Build history of the part. All positions in model axes, mm. A direction names the side the tool comes from. Round coordinates to 2 decimals unless told otherwise and drop trailing zeros. Order: outer loops, then holes, each group sorted by start corner. A loop starts at its lowest first (then second) coordinate and runs counter-clockwise, first axis right, second up. Notation, with made-up numbers: (80.25, -35.75) -> (125.25, -35.75) arc R26 ccw to (125.25, -12.75) -> close; hole circle Ø7 at (-5, 45.25). An arc over 180 degrees is marked (long way). Answer as a JSON object with one key per item and string values.
from build123d import *

# Parameters (mm, degrees)
BOSS_EXTRUDE1_DEPTH = 24
BOSS_EXTRUDE2_DEPTH = 5
CHAMFER1_SIZE       = 8.038475773
CHAMFER1_SIZE_2     = 30
FILLET1_R           = 20
SKETCH3_W           = 4.2
SKETCH3_H           = 4.2
BOSS_EXTRUDE3_DEPTH = 10


with BuildPart() as part:
    # Sketch1 → Boss-Extrude1 (new body)
    with BuildSketch(Plane(origin=(0, 0, 0), x_dir=(1, 0, 0), z_dir=(0, 1, 0))):
        with BuildLine():
            Line((0, 28), (0, 18))
            ThreePointArc((0, 18), (18, 0), (0, -18))
            Line((0, -18), (0, -28))
            ThreePointArc((0, -28), (28, 0), (0, 28))
        make_face()
    extrude(amount=BOSS_EXTRUDE1_DEPTH)

    # Sketch2 → Boss-Extrude2 (add)
    with BuildSketch(Plane(origin=(0, 24, 0), x_dir=(1, 0, 0), z_dir=(0, 1, 0))):
        with BuildLine():
            Line((0, 28), (0, 15.5))
            ThreePointArc((0, 15.5), (15.5, 0), (0, -15.5))
            Line((0, -15.5), (0, -28))
            ThreePointArc((0, -28), (28, 0), (0, 28))
        make_face()
    extrude(amount=BOSS_EXTRUDE2_DEPTH)

    # Chamfer1
    # the kernel refuses this chamfer: 30, 8.038475773 mm, written as the material it takes off along each edge
    with BuildSketch(Plane(origin=(0, 29, 0), x_dir=(-0.9999950652018581, 0, 0.0031415874858793337), z_dir=(-0.0031415874858793337, 0, -0.9999950652018581))) as chamfer1_piece_1:
        Polygon((28 - CHAMFER1_SIZE, 0), (28, -CHAMFER1_SIZE_2), (28, 0), align=None)
    revolve(axis=Axis((0, 29, 0), (0, 1, 0)), revolution_arc=359.64, mode=Mode.SUBTRACT)

    # Fillet1
    # the kernel refuses this fillet: 20 mm, written as the material it takes off along each edge
    with BuildSketch(Plane(origin=(0, 29, 0), x_dir=(-0.9872402067146837, 0, 0.1592381055085398), z_dir=(-0.1592381055085398, 0, -0.9872402067146837))) as fillet1_piece_1:
        with BuildLine():
            CenterArc((3.55400198, -16.040359451), FILLET1_R, 15, 38.323238927)
            Line((15.5, 0), (15.73891996, 0.320807189))
            ThreePointArc((15.73891996, 0.320807189), (17.730762114, 0.4), (19.961524227, 0.4))
            Line((19.961524227, 0.4), (20.347894558, 0.103527618))
            Line((20.347894558, 0.103527618), (23.258888836, -10.76045093))
            Line((23.258888836, -10.76045093), (22.872518506, -10.863978548))
        make_face()
    revolve(axis=Axis((0, 29, 0), (0, 1, 0)), revolution_arc=341.674648162, mode=Mode.SUBTRACT)

    # Sketch3 → Boss-Extrude3 (add)
    with BuildSketch(Plane.ZY):
        with Locations((21.5, 4.1)):
            Rectangle(SKETCH3_W, SKETCH3_H)
        with Locations((-21.5, 4.1)):
            Rectangle(SKETCH3_W, SKETCH3_H)
    extrude(amount=BOSS_EXTRUDE3_DEPTH)


solid = part.part
1) Cut at A-A, the plane y = 5. Give the cut face in (x, z), plus the area to 3 significant figures.
Checked values:
{"outline": "(-10, -23.6) -> (0, -23.6) -> (0, -26.39) arc R26.39 ccw to (0, 26.39) -> (0, 23.6) -> (-10, 23.6) -> (-10, 19.4) -> (0, 19.4) -> (0, 18) arc R18 cw to (0, -18) -> (0, -19.4) -> (-10, -19.4) -> close", "area": "669 mm²"}
2) Pull direction Z, two halves, no side cores. Call faces 6 (the face through (-5, 4, -23.6)), 7 (the face through (18, 12, 0)), 8 (the face through (-10, 4, 21)): pulls with the +Z half, pulls with the -Z half, needs draft (parallel to the pull), parting line crosses it, or undercut.
Checked values:
{"face 6": "pulls with the -Z half", "face 7": "undercut", "face 8": "needs draft"}
3) Flat gauge pins, fed straight in: pin 1 Ø2 at (x, y) = (-4, 3.5) entering from +Z; pin 2 Ø8 at (y, z) = (7, -7) entering from +X; pin 3 Ø2 at (x, z) = (-5, 22) entering from -Y. Where does each tip first touch, or does it go through?
Checked values:
{"pin 1": "stops at z = 23.6", "pin 2": "stops at x = 26.32", "pin 3": "stops at y = 2"}
4) Probe L1, parallel to Z at x = 14, y = 2.75; L2, parallel to Z at x = 14, y = 25.75; L3, parallel to Y at x = 5, z = -15. List the from-to ranges inside material, lowest first. Write a range as from..to.
Checked values:
{"L1": "z = -23.08..-11.31, 11.31..23.08", "L2": "z = -12.74..-6.65, 6.65..12.74", "L3": "y = 24..28.76"}
5) Cut at B-B, the plane y = 11.25. Give the cut face in (x, z).
Checked values:
{"outline": "(0, -24.72) arc R24.72 ccw to (0, 24.72) -> (0, 18) arc R18 cw to (0, -18) -> close"}
6) Cut at C-C, the plane y = 16.5. Give the cut face in (x, z), plus the area to 3 significant figures.
Checked values:
{"outline": "(0, -23.31) arc R23.31 ccw to (0, 23.31) -> (0, 18) arc R18 cw to (0, -18) -> close", "area": "345 mm²"}
7) Which spindle directions (+Z, -Z, +X, -X, +Y, -Y) get a long thin tool onto all of the face, cutting with end or side? Do faces 1 (the face through (-5, 6.2, 21)), 2 (the face through (16, 24, -1)), 3 (the face through (-5, 2, -22)), 4 (the face through (-5, 4, -19.4)), 5 (the face through (-5, 4, 23.6)). Say none if no direction does.
Checked values:
{"face 1": "+Z, -Z, -X, +Y", "face 2": "-X, -Y", "face 3": "+Z, -Z, -X, -Y", "face 4": "-X, +Y, -Y", "face 5": "+Z, -X, +Y, -Y"}
